```python
from build123d import *

# Parameters (mm, degrees)
SKETCH1_W           = 6.35
SKETCH1_H           = 40.5892
BOSS_EXTRUDE1_DEPTH = 3.4036


with BuildPart() as part:
    # Sketch1 → Boss-Extrude1 (new body)
    with BuildSketch(Plane.XY):
        Polygon((8565.704586486, 2936.318079168), (8660.954586486, 2933.984454168), (8660.954586486, 2933.828879168), (8972.104586486, 2933.828879168), (8972.104586486, 2921.128879168), (8965.754586486, 2921.128879168), (8965.754586486, 2880.539679168), (8972.104586486, 2880.539679168), (8972.104586486, 2867.839679168), (8660.954586486, 2867.839679168), (8660.954586486, 2867.684104168), (8565.704586486, 2865.350479168), (8565.704586486, 2878.050479168), (8572.054586486, 2878.050479168), (8572.054586486, 2923.618079168), (8565.704586486, 2923.618079168), align=None)
        with Locations((8664.129586486, 2900.834279168)):
            Rectangle(SKETCH1_W, SKETCH1_H, mode=Mode.SUBTRACT)
        with BuildLine():
            Line((8683.179586486, 2890.064679168), (8683.179586486, 2911.603879168))
            ThreePointArc((8683.179586486, 2911.603879168), (8685.039458425, 2916.094007229), (8689.529586486, 2917.953879168))
            Line((8689.529586486, 2917.953879168), (8784.779586486, 2917.953879168))
            ThreePointArc((8784.779586486, 2917.953879168), (8789.269714547, 2916.094007229), (8791.129586486, 2911.603879168))
            Line((8791.129586486, 2911.603879168), (8791.129586486, 2890.064679168))
            ThreePointArc((8791.129586486, 2890.064679168), (8789.269714547, 2885.574551108), (8784.779586486, 2883.714679168))
            Line((8784.779586486, 2883.714679168), (8689.529586486, 2883.714679168))
            ThreePointArc((8689.529586486, 2883.714679168), (8685.039458425, 2885.574551108), (8683.179586486, 2890.064679168))
        make_face(mode=Mode.SUBTRACT)
        with BuildLine():
            Line((8648.254586486, 2911.603879168), (8648.254586486, 2890.064679168))
            ThreePointArc((8648.254586486, 2890.064679168), (8646.394714547, 2885.574551108), (8641.904586486, 2883.714679168))
            Line((8641.904586486, 2883.714679168), (8591.104586486, 2883.714679168))
            ThreePointArc((8591.104586486, 2883.714679168), (8586.614458425, 2885.574551108), (8584.754586486, 2890.064679168))
            Line((8584.754586486, 2890.064679168), (8584.754586486, 2911.603879168))
            ThreePointArc((8584.754586486, 2911.603879168), (8586.614458425, 2916.094007229), (8591.104586486, 2917.953879168))
            Line((8591.104586486, 2917.953879168), (8641.904586486, 2917.953879168))
            ThreePointArc((8641.904586486, 2917.953879168), (8646.394714547, 2916.094007229), (8648.254586486, 2911.603879168))
        make_face(mode=Mode.SUBTRACT)
        with BuildLine():
            Line((8943.529586486, 2917.953879168), (8835.579586486, 2917.953879168))
            ThreePointArc((8835.579586486, 2917.953879168), (8831.089458425, 2916.094007229), (8829.229586486, 2911.603879168))
            Line((8829.229586486, 2911.603879168), (8829.229586486, 2890.064679168))
            ThreePointArc((8829.229586486, 2890.064679168), (8831.089458425, 2885.574551108), (8835.579586486, 2883.714679168))
            Line((8835.579586486, 2883.714679168), (8943.529586486, 2883.714679168))
            ThreePointArc((8943.529586486, 2883.714679168), (8948.019714547, 2885.574551108), (8949.879586486, 2890.064679168))
            Line((8949.879586486, 2890.064679168), (8949.879586486, 2911.603879168))
            ThreePointArc((8949.879586486, 2911.603879168), (8948.019714547, 2916.094007229), (8943.529586486, 2917.953879168))
        make_face(mode=Mode.SUBTRACT)
        with Locations((8810.179586486, 2900.834279168)):
            Rectangle(SKETCH1_W, SKETCH1_H, mode=Mode.SUBTRACT)
    extrude(amount=BOSS_EXTRUDE1_DEPTH)


solid = part.part
```
For this review, take the finished solid that the model builds, in its own axes (mm). A direction names the side the tool comes from. Round coordinates to 2 decimals unless told otherwise and drop trailing zeros. Write each loop counter-clockwise with the first axis right and the second up, starting at its lowest first coordinate (ties: lowest second). Pieces come first, ordered by that corner, then holes. Notation, with made-up numbers: (16, -12) -> (23, -12) arc R33 cw to (23, 23) -> close; hole circle Ø6 at (80.5, 27.25). An arc over 180 degrees is marked (long way). Use one line per item in the form item = value.
1) To check wall thickness, follow L1, parallel to X at y = 2904, z = 1; L2, parallel to X at y = 2881.5, z = 1.7; L3, parallel to X at y = 2917, z = 1.7. State the ranges of each line that lie inside material, in increasing order. Write a range as from..to.
Found:
L1 = 8572.05..8584.75, 8648.25..8660.95, 8667.3..8683.18, 8791.13..8807, 8813.35..8829.23, 8949.88..8965.75
L2 = 8572.05..8660.95, 8667.3..8807, 8813.35..8965.75
L3 = 8572.05..8587.76, 8645.25..8660.95, 8667.3..8686.18, 8788.13..8807, 8813.35..8832.23, 8946.88..8965.75
2) Tool access review of faces 1 (the flat face through (8772, 2925, 3.404)), 2 (the cylindrical face through (8831, 2916, 2)): name each direction out of +Z, -Z, +X, -X, +Y, -Y from which nothing blocks a thin tool from reaching the whole face with its end or side.
Found:
face_1 = +Z, +X, -X, +Y, -Y
face_2 = +Z, -Z
3) Take a section at C-C, the plane x = 8673. Write out the cut boundary in (y, z), and give its area (3 significant figures).
Found:
outline = (2867.84, 0) -> (2933.83, 0) -> (2933.83, 3.4) -> (2867.84, 3.4) -> close
area = 225 mm2
4) Take a section at A-A, the plane x = 8886.5. Write out the cut boundary in (y, z).
Found:
outline = (2867.84, 0) -> (2883.71, 0) -> (2883.71, 3.4) -> (2867.84, 3.4) -> close; (2917.95, 0) -> (2933.83, 0) -> (2933.83, 3.4) -> (2917.95, 3.4) -> close
5) Mouldability with a two-part tool opening along X and no side actions: class faces 3 (the flat face through (8772, 2925, 0)), 4 (the cylindrical face through (8685.089, 2885.525, 1.678)) as +X half, -X half, draft (parallel to the pull), parting line (faces both ways), or undercut.
Found:
face_3 = draft
face_4 = undercut
6) Clearance check with flat-ended pins moving along their axes: pin 1 (1 mm diameter, centred on x = 8627.5, z = 1, fed in from +Y); pin 2 (2 mm diameter, centred on x = 8893, z = 1, fed in from -Y); pin 3 (1 mm diameter, centred on y = 2898.5, z = 2.5, fed in from +X). State where each tip first meets the part, or that it passes through.
Found:
pin_1 = 2934.82
pin_2 = 2867.84
pin_3 = 8965.75
7) Take a section at B-B, the plane z = 0.8. Count the separate pieces of the cut face and the enclosed holes in it, and give its area (3 significant figures).
Found:
separate_pieces = 1
enclosed_holes = 5
area = 16,100 mm2
